from build123d import *

# Parameters (mm, degrees)
F0_W      = 42.5921405452
F0_H      = 76.2
F1_DEPTH  = 19.05
F2_R      = 5.08
F3_R      = 7.4390090137
F4_DEPTH  = 25.4
F8_DEPTH  = 10.16
F9_R      = 5.08
F10_R     = 5.4254130452
F11_DEPTH = 25.4
F12_SIZE  = 1.27


with BuildPart() as f1:
    # F0 (on Front) → F1 (new body)
    with BuildSketch(Plane.XZ):
        Rectangle(F0_W, F0_H)
    extrude(amount=F1_DEPTH)

    # F2
    f2_edges = [f1.edges().sort_by_distance(p)[0] for p in [
        (-21.29607, -9.525, 38.1),
        (21.29607, -9.525, 38.1),
        (21.29607, -9.525, -38.1),
        (-21.29607, -9.525, -38.1),
    ]]
    fillet(f2_edges, radius=F2_R)

    # F3 (on face) → F4 (cut)
    with BuildSketch(Plane.XZ.offset(19.05)):
        with Locations((-10.371832177, -23.3288127929)):
            Circle(F3_R)
        with BuildLine():
            Line((8.7983496487, 31.6190682352), (-8.7983496487, 31.6190682352))
            ThreePointArc((-8.7983496487, 31.6190682352), (-15.4311150855, 24.9863027984), (-8.7983496487, 18.3535373615))
            Line((-8.7983496487, 18.3535373615), (8.7983496487, 18.3535373615))
            ThreePointArc((8.7983496487, 18.3535373615), (15.4311150855, 24.9863027984), (8.7983496487, 31.6190682352))
        make_face()
    extrude(amount=-F4_DEPTH, mode=Mode.SUBTRACT)

    # F7 (on face) → F8 (join, symmetric)
    with BuildSketch(Plane(origin=(1.5022693661, 0, -1.79863414), x_dir=(0.7675056841, 0, 0.6410421397), z_dir=(0.6410421397, 0, -0.7675056841))):
        Polygon((0.1007605708, 19.05), (8.8891370815, 19.05), (24.1558142006, 44.8086634278), (17.6520292383, 48.6633348998), align=None)
    extrude(amount=F8_DEPTH, both=True)

    # F9
    f9_edges = [f1.edges().sort_by_distance(p)[0] for p in [
        (11.03316, -46.735999, 19.399518),
        (24.059136, -46.735999, 3.803803),
    ]]
    fillet(f9_edges, radius=F9_R)

    # F10 (on face) → F11 (cut)
    with BuildSketch(Plane(origin=(-6.3556814341, -4.907967933, -5.3084422822), x_dir=(0.3913195596, -0.860258078, 0.3268410032), z_dir=(-0.6602529647, -0.5098588424, -0.551461679))):
        with Locations((41.8185740709, -1.9313164521)):
            Circle(F10_R)
    extrude(amount=-F11_DEPTH, mode=Mode.SUBTRACT)

    # F12
    f12_edges = [f1.edges().sort_by_distance(p)[0] for p in [
        (-21.29607, -19.05, 0),
        (-21.29607, 0, 0),
    ]]
    chamfer(f12_edges, length=F12_SIZE)


solid = f1.part
Input: part model. Units: mm. Frame: model coordinates. A direction names the side the tool comes from. Round coordinates to 2 decimals unless told otherwise and drop trailing zeros. Loops run counter-clockwise (first coordinate to the right, second up) from the corner with the lowest first, then second, coordinate; pieces in that order, holes last. Notation, with made-up numbers: (4.5, 64) -> (18.5, 64) arc R25 cw to (18.5, 90) -> close; hole circle Ø1 at (82.25, 17.5). An arc over 180 degrees is marked (long way). Answer as a JSON object with one key per item and string values. Group by question number.
1) Section query B-B on x = -13. Output: boundary loops of the cut face in (y, z).
2) Draft query along X for faces 1 (the cylindrical face through (11.33, -45.45, 17.76)), 2 (the flat face through (14.19, -31.75, 8.62)), 3 (the cylindrical face through (15.43, -9.66, 24.84)). Return one class per face: +X half, -X half, draft (parallel to the pull), parting line (faces both ways), or undercut.
3) Pin query (flat end, axial travel): pin 1 (5 mm diameter, centred on x = 12.5, z = -26.5, fed in from -Y); pin 2 (12 mm diameter, centred on x = 15, y = -26.5, fed in from -Z); pin 3 (10 mm diameter, centred on y = -26, z = -4.5, fed in from -X). Return the tip coordinate at first contact, or that it passes through.
4) Section query D-D on x = -7. Output: boundary loops of the cut face in (y, z), plus the area to 3 significant figures.
5) Reachability of faces 4 (the cylindrical face through (22.5, -45.45, 4.39)), 5 (the flat face through (3.19, -31.85, 12.85)), 6 (the flat face through (0, -10, 31.619)) from +Z, -Z, +X, -X, +Y, -Y: full face, straight path, thin tool, end or side. Return the list, or none.
6) Ray query, L1, parallel to Z at x = 7.5, y = -2.5; L2, parallel to Y at x = -18, z = -24; L3, parallel to Y at x = 11, z = 7.5. Return the intervals inside material, ascending.
7) Section query A-A on z = 29. Output: boundary loops of the cut face in (x, y), plus the area to 3 significant figures.
8) Section query C-C on y = -16. Output: boundary loops of the cut face in (x, z), plus the area to 3 significant figures.
Reply:
{
 "1": {"outline": "(-19.05, -36.83) -> (-17.78, -38.1) -> (-1.27, -38.1) -> (0, -36.83) -> (0, -30.29) -> (-19.05, -30.29) -> close; (-19.05, -16.37) -> (0, -16.37) -> (0, 19.85) -> (-19.05, 19.85) -> close; (-19.05, 30.12) -> (0, 30.12) -> (0, 36.83) -> (-1.27, 38.1) -> (-17.78, 38.1) -> (-19.05, 36.83) -> close"},
 "2": {"face 1": "parting line", "face 2": "+X half", "face 3": "undercut"},
 "3": {"pin 1": "stops at y = -19.05", "pin 2": "stops at z = -7.95", "pin 3": "stops at x = 3.57"},
 "4": {"outline": "(-19.05, -36.83) -> (-17.78, -38.1) -> (-1.27, -38.1) -> (0, -36.83) -> (0, -29.96) -> (-19.05, -29.96) -> close; (-19.05, -16.7) -> (0, -16.7) -> (0, 18.35) -> (-19.05, 18.35) -> close; (-19.05, 31.62) -> (0, 31.62) -> (0, 36.83) -> (-1.27, 38.1) -> (-17.78, 38.1) -> (-19.05, 36.83) -> close", "area": "943 mm2"},
 "5": {"face 4": "+X, -Y", "face 5": "+Z, -X, -Y", "face 6": "+Y, -Y"},
 "6": {"L1": "z = -38.1 to 18.35, 31.62 to 38.1", "L2": "y = -19.05 to 0", "L3": "y = -34.5 to -26.41, -19.05 to 0"},
 "7": {"outline": "(-21.3, -17.78) -> (-20.03, -19.05) -> (-14.08, -19.05) -> (-14.08, 0) -> (-20.03, 0) -> (-21.3, -1.27) -> close; (14.08, -19.05) -> (20.03, -19.05) -> (21.3, -17.78) -> (21.3, -1.27) -> (20.03, 0) -> (14.08, 0) -> close", "area": "272 mm2"},
 "8": {"outline": "(-21.3, -33.02) arc R5.08 ccw to (-16.22, -38.1) -> (16.22, -38.1) arc R5.08 ccw to (21.3, -33.02) -> (21.3, 33.02) arc R5.08 ccw to (16.22, 38.1) -> (-16.22, 38.1) arc R5.08 ccw to (-21.3, 33.02) -> close; hole circle Ø14.88 at (-10.37, -23.33); hole (-8.8, 18.35) -> (8.8, 18.35) arc R6.63 ccw to (8.8, 31.62) -> (-8.8, 31.62) arc R6.63 ccw to start", "area": "2,680 mm2"}
}
